CAD build for the part. Positions are in the model's coordinates, mm. Face numbers are marked on the shaded views. Give positions to 0.01 mm unless a question says otherwise; leave off trailing zeros. Write each loop counter-clockwise with the first axis right and the second up, starting at its lowest first coordinate (ties: lowest second). Pieces come first, ordered by that corner, then holes. Notation, with made-up numbers: (77, -9.5) - (125, -9.5) arc R27 ccw to (125, 29.5) - close; hole circle Ø1 at (-14.5, -34). An arc over 180 degrees is marked (long way). Answer as a JSON object with one key per item and string values.
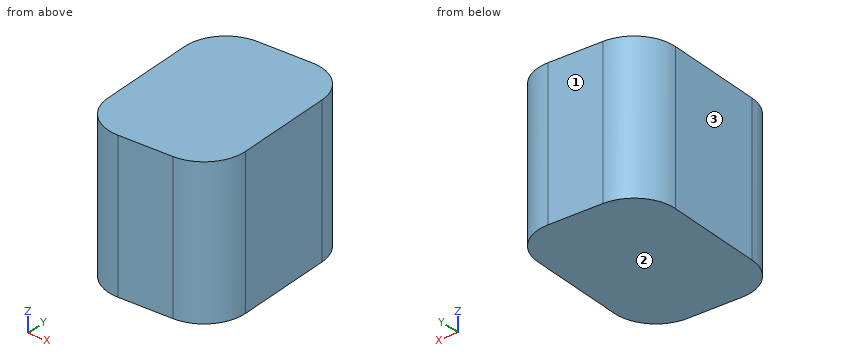
Autodesk Inventor part; units mm, degrees
ref_plane "Work Plane1" through (-89.0919, -102.1665, 32.7858) normal (0, 0, -1) x (0, 1, 0)
ref_plane "YZ Plane" through (0, 0, 0) normal (1, 0, 0) x (0, 1, 0)
ref_plane "XZ Plane" through (0, 0, 0) normal (0, 1, 0) x (-1, 0, 0)
sketch "Sketch1" plane through (0, 0, 0) normal (0, 0, 1) x (1, 0, 0)
  circle A0 centre (9.0867, 110.4972) radius 1.6
  arc A1 (10.396, 90.5401) -> (7.7775, 130.4543) centre (9.0867, 110.4972) ccw
  line L0 (-242.3149, 114.047) -> (7.7775, 130.4543)
  line L1 (-239.6964, 74.1328) -> (-242.3149, 114.047)
  line L2 (10.396, 90.5401) -> (-239.6964, 74.1328)
  circle A2 centre (9.0867, 110.4972) radius 20
  line L3 (-242.3149, 114.047) -> (-212.3793, 116.0109)
  line L4 (-212.3793, 116.0109) -> (-209.7607, 76.0967)
  point P0 (0, 0)
  dimension "d0" = 30
ref_plane "Work Plane1" through (-89.0919, -102.1665, 32.7858) normal (0, 0, -1) x (0, 1, 0)
extrude "Extrusion1" add sketch "Sketch1" along normal up to surface (32.7858 mm away) contours L2 L1 L0 L4
fillet "Fillet1" radius 9 4 edges at (-209.7607, 76.0967, 16.3929) (-239.6964, 74.1328, 16.3929) (-212.3793, 116.0109, 16.3929) (-242.3149, 114.047, 16.3929)
properties part number "wspornik"
(1) Saw through at C-C, the plane y = 113. Give the cut face in (x, z).
Answer key:
{"outline": "(-237.95, 0) - (-214.61, 0) - (-214.61, 32.79) - (-237.95, 32.79) - close"}
(2) Flat gauge pins, fed straight in: P1, Ø8, axis at y = 103.5, z = 14, coming from the +X side; P2, Ø5, axis at y = 98, z = 26, coming from the -X side; P3, Ø10, axis at y = 96.5, z = 19, coming from the +X side. Where does each tip first touch, or does it go through?
Answer key:
{"P1": "stops at x = -211.3", "P2": "stops at x = -241.43", "P3": "stops at x = -210.77"}
(3) Saw through at A-A, the plane z = 5. Give the cut face in (x, y), and give its area (3 significant figures).
Answer key:
{"outline": "(-241.73, 105.07) - (-240.29, 83.11) arc R9 ccw to (-230.72, 74.72) - (-218.74, 75.51) arc R9 ccw to (-210.35, 85.08) - (-211.79, 107.03) arc R9 ccw to (-221.36, 115.42) - (-233.33, 114.64) arc R9 ccw to start", "area": "1,130 mm²"}
(4) Saw through at B-B, the plane x = -222. Give the cut face in (y, z).
Answer key:
{"outline": "(75.29, 0) - (115.38, 0) - (115.38, 32.79) - (75.29, 32.79) - close"}
(5) Pull direction Y, two halves, no side cores. Call the marked faces 1, 2 and 3: pulls with the +Y half, pulls with the -Y half, needs draft (parallel to the pull), parting line crosses it, or undercut.
Answer key:
{"face 1": "pulls with the +Y half", "face 2": "needs draft", "face 3": "pulls with the -Y half"}
(6) Probe L1, parallel to Y at x = -219.5, z = 27; L2, parallel to X at y = 96.5, z = 25; L3, parallel to X at y = 92, z = 29. List the from-to ranges inside material, lowest first. Write a range as [from, to].
Answer key:
{"L1": "y = [75.46, 115.35]", "L2": "x = [-241.16, -211.1]", "L3": "x = [-240.87, -210.8]"}
